Autodesk Inventor part; units mm, degrees
ref_plane "YZ Plane" through (0, 0, 0) normal (1, 0, 0) x (0, 1, 0)
ref_plane "XZ Plane" through (0, 0, 0) normal (0, 1, 0) x (-1, 0, 0)
ref_plane "XY Plane" through (0, 0, 0) normal (0, 0, 1) x (1, 0, 0)
sketch "Sketch1" plane through (0, 0, 0) normal (1, 0, 0) x (0, 1, 0)
  line L0 (30, 0) -> (0, 0)
  line L1 (0, 0) -> (0, -14)
  line L2 (0, -14) -> (4, -14)
  line L3 (4, -14) -> (4, -3)
  line L4 (4, -3) -> (30, -3)
  line L5 (30, -3) -> (30, 0)
  dimension "d0" = 4
  dimension "d1" = 14
  dimension "d2" = 3
  dimension "d3" = 30
extrude "Extrusion1" add sketch "Sketch1" against normal mid plane 15
sketch "Sketch2" plane through (-7.5, 4, -14) normal (0, 1, 0) x (1, 0, 0)
  circle A0 centre (7.5, -7.5) radius 1.25
  line L0 (0, 0) -> (15, 0)
  line L1 (0, -14) -> (15, -14)
  line L2 (0, -11) -> (15, -11)
  point P0 (7.5, -14)
  point P1 (7.5, -14)
  dimension "d6" = 2.5
  dimension "d10" = 3.5
extrude "Extrusion2" cut sketch "Sketch2" against normal through all
properties part number "battery_fix_board"
Design review of the part built by this model. Coordinates are the model's own, in mm. A direction names the side the tool comes from. Give positions to 0.01 mm unless a question says otherwise; leave off trailing zeros. Order: outer loops, then holes, each group sorted by start corner. A loop starts at its lowest first (then second) coordinate and runs counter-clockwise, first axis right, second up. Notation, with made-up numbers: (13.5, 62) -> (40.5, 62) arc R24 ccw to (40.5, 95) -> close; hole circle Ø9 at (-32.5, -2). An arc over 180 degrees is marked (long way). Write item = value, one per line. Start each with the question number.
(1) We need section C-C on z = -11.5. Write out the cut boundary in (x, y), plus the area to 3 significant figures.
(2) We need section A-A on z = -6.5. Write out the cut boundary in (x, y).
(3) Mouldability with a two-part tool opening along X and no side actions: class faces 1 (the face through (0, 0, -8)), 2 (the face through (-7.5, 9.4, -2.8)), 3 (the face through (-0.27, 2.03, -5.28)) as +X half, -X half, draft (parallel to the pull), parting line (faces both ways), or undercut.
(4) For pin 1 (1.5 mm diameter, centred on x = 4, y = 14, fed in from +Z); pin 2 (6 mm diameter, centred on x = -5, y = 10.5, fed in from -Z), all flat-tipped, find the tip position at first contact; note any pin that passes through.
(5) We need section B-B on x = 0. Write out the cut boundary in (y, z).
(6) We need section D-D on x = -5. Write out the cut boundary in (y, z).
(7) For faces 4 (the face through (7.5, 9.4, -2.8)), 5 (the face through (0, 17, -3)), list the 3-axis set-ups (+Z, -Z, +X, -X, +Y, -Y) from which the entire face can be reached by the end or side of a thin tool; tool diameter is ignored.
(8) To check wall thickness, follow line 1 along Z through (x, y) = (0, 1.3); line 2 along X through (y, z) = (1.15, -6.5); line 3 along Z through (x, y) = (-0.5, 15.5). State the ranges of each line that lie inside material, in increasing order.
Numbers:
q1.outline = (-7.5, 0) -> (7.5, 0) -> (7.5, 4) -> (-7.5, 4) -> close
q1.area = 60.0 mm^2
q2.outline = (-7.5, 0) -> (-1.25, 0) -> (-1.25, 4) -> (-7.5, 4) -> close; (1.25, 0) -> (7.5, 0) -> (7.5, 4) -> (1.25, 4) -> close
q3.face_1 = draft
q3.face_2 = -X half
q3.face_3 = undercut
q4.pin_1 = 0
q4.pin_2 = -3
q5.outline = (0, -14) -> (4, -14) -> (4, -7.75) -> (0, -7.75) -> close; (0, -5.25) -> (4, -5.25) -> (4, -3) -> (30, -3) -> (30, 0) -> (0, 0) -> close
q6.outline = (0, -14) -> (4, -14) -> (4, -3) -> (30, -3) -> (30, 0) -> (0, 0) -> close
q7.face_4 = +Z, -Z, +X, +Y, -Y
q7.face_5 = -Z, +X, -X, +Y
q8.line_1 = -14 to -7.75, -5.25 to 0
q8.line_2 = -7.5 to -1.25, 1.25 to 7.5
q8.line_3 = -3 to 0
